Part print with two shaded views. Sizes in mm from the minimum x, y, z corner. A direction names the side the tool comes from. Round coordinates to 2 decimals unless told otherwise and drop trailing zeros. Write each loop counter-clockwise with the first axis right and the second up, starting at its lowest first coordinate (ties: lowest second). Pieces come first, ordered by that corner, then holes. Notation, with made-up numbers: (43.5, 14) -> (52.5, 14) arc R15 ccw to (52.5, 29) -> close; hole circle Ø8 at (67, -14). An arc over 180 degrees is marked (long way). Answer as CSV lines item,"result".
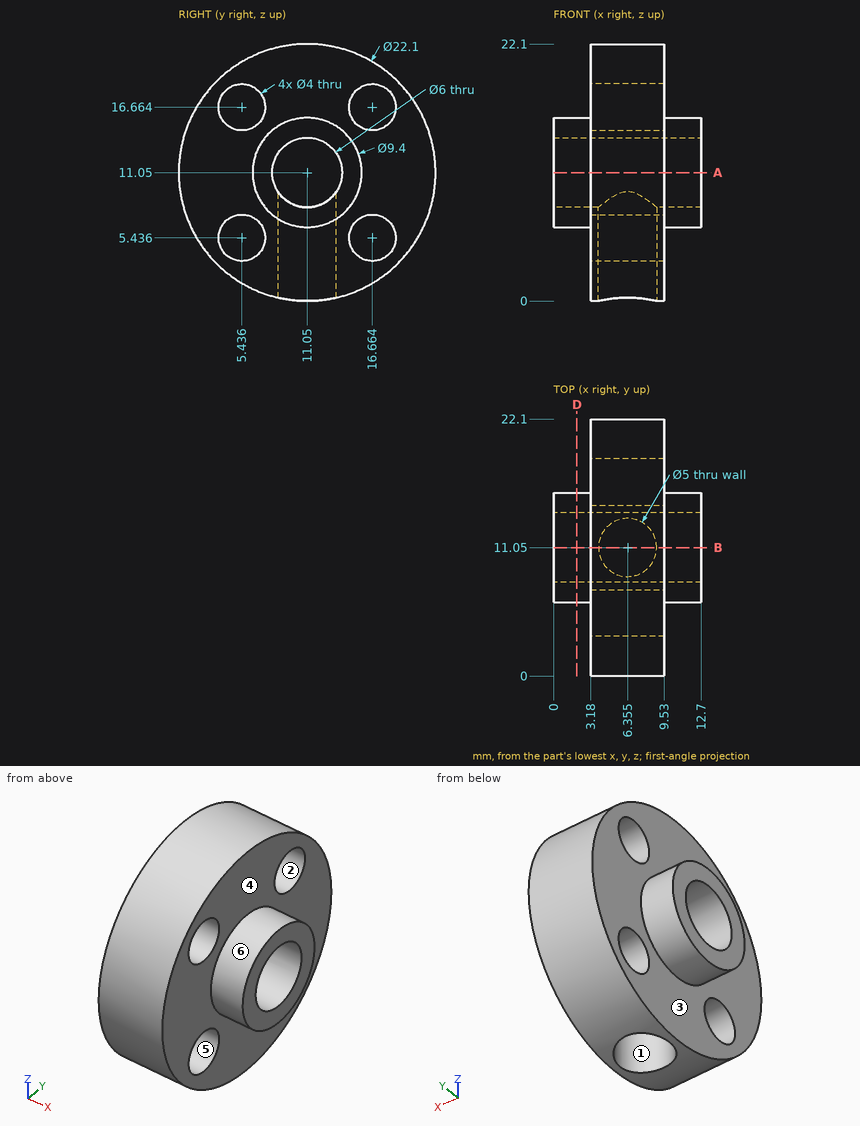
1. Cut at A-A, the plane z = 11.05. Write the cut outline in (x, y).
Results found:
outline,"(0, 6.35) -> (3.18, 6.35) -> (3.18, 0) -> (9.53, 0) -> (9.53, 6.35) -> (12.7, 6.35) -> (12.7, 8.05) -> (0, 8.05) -> close; (0, 14.05) -> (12.7, 14.05) -> (12.7, 15.75) -> (9.53, 15.75) -> (9.53, 22.1) -> (3.18, 22.1) -> (3.18, 15.75) -> (0, 15.75) -> close"
2. Drop flat-ended pins along their axis: pin 1 Ø6.5 at (y, z) = (15, 15) entering from -X; pin 2 Ø4.5 at (y, z) = (16.66, 5.44) entering from +X; pin 3 Ø2 at (x, z) = (8, 6) entering from -Y; pin 4 Ø1.5 at (x, y) = (2, 5) entering from -Z. Give the stop position or say it passes through.
Results found:
pin 1,"stops at x = 0"
pin 2,"stops at x = 9.53"
pin 3,"stops at y = 0.77"
pin 4,"passes through"
3. Cut at B-B, the plane y = 11.05. Count the separate pieces of the cut face and the enclosed holes in it.
Results found:
separate pieces,"3"
enclosed holes,"0"
4. Which spindle directions (+Z, -Z, +X, -X, +Y, -Y) get a long thin tool onto all of the face, cutting with end or side? Do the marked faces 1, 2 and 3. Say none if no direction does.
Results found:
face 1,"-Z"
face 2,"+X, -X"
face 3,"-X"
5. Mould opens along Z. For the marked faces 4, 5 and 6 say: +Z half, -Z half, draft (parallel to the pull), parting line (faces both ways), or undercut.
Results found:
face 4,"draft"
face 5,"undercut"
face 6,"parting line"
6. Probe line 1 along Y through (x, z) = (1.5, 11); line 2 along Z through (x, y) = (1.5, 11.25) (1 decimal); line 3 along Y through (x, z) = (6.75, 11.05). List the from-to ranges inside material, lowest first.
Results found:
line 1,"y = 6.35 to 8.05, 14.05 to 15.75"
line 2,"z = 6.4 to 8.1, 14 to 15.7"
line 3,"y = 0 to 8.05, 14.05 to 22.1"
7. Cut at D-D, the plane x = 2. Write the cut outline in (y, z).
Results found:
outline,"circle Ø9.4 at (11.05, 11.05); hole circle Ø6 at (11.05, 11.05)"
